The model under review builds one solid part; all positions refer to its coordinate system, in mm. A direction names the side the tool comes from. Coordinates: 2 decimals unless noted, no trailing zeros. Order: outer loops, then holes, each group sorted by start corner. A loop starts at its lowest first (then second) coordinate and runs counter-clockwise, first axis right, second up. Notation, with made-up numbers: (-18.5, 31.5) - (29.5, 31.5) arc R12 ccw to (29.5, 46.5) - close; hole circle Ø11 at (81, -3). An arc over 180 degrees is marked (long way). Answer in a Markdown table with one row per item.
```python
from build123d import *

# Parameters (mm, degrees)
F1_DEPTH  = 1
F4_W      = 25.4
F4_H      = 50.8
F5_DEPTH  = 34
F6_W      = 1.778
F6_H      = 3.81
F7_DEPTH  = 17.78
F8_W      = 20.32
F8_H      = 12.7
F9_DEPTH  = 7.62
F11_DEPTH = 25.4


with BuildPart() as f1:
    # F0 (on Top) → F1 (new body)
    with BuildSketch(Plane.XY):
        Polygon((12.7, 30), (0, 30), (0, 0), (20, 0), align=None)
    extrude(amount=F1_DEPTH)

    # F2: F1 across plane


with BuildPart() as f1_1:
    add(f1.part)
    add(f1.part.mirror(Plane.XZ))

    # F3: F1 across plane


with BuildPart() as f1_2:
    add(f1_1.part)
    add(f1_1.part.mirror(Plane.YZ))

    # F4 (on face) → F5 (join)
    with BuildSketch(Plane.XY.offset(1)):
        with Locations((-0.045811, 0)):
            Rectangle(F4_W, F4_H)
    extrude(amount=F5_DEPTH)

    # F6 (on face) → F7 (cut)
    with BuildSketch(Plane(origin=(0, 0, 0), x_dir=(1, 0, 0), z_dir=(0, 0, -1))):
        Polygon((-5.4, -22.54), (5, -22.54), (12.3, -15.24), (12.3, -2.54), (-12.7, -2.54), (-12.7, -15.24), align=None)
        with Locations((-5.969, -9.508814)):
            Rectangle(F6_W, F6_H, mode=Mode.SUBTRACT)
        with Locations((0.038805, -15.194196)):
            Rectangle(F6_W, F6_H, mode=Mode.SUBTRACT)
        with Locations((5.969, -9.508814)):
            Rectangle(F6_W, F6_H, mode=Mode.SUBTRACT)
    extrude(amount=-F7_DEPTH, mode=Mode.SUBTRACT)

    # F8 (on face) → F9 (join)
    with BuildSketch(Plane(origin=(0, 0, 0), x_dir=(1, 0, 0), z_dir=(0, 0, -1))):
        with Locations((0, 14.463713)):
            Rectangle(F8_W, F8_H)
    extrude(amount=F9_DEPTH)

    # F10 (on face) → F11 (cut)
    with BuildSketch(Plane(origin=(0, -8.113713, 0), x_dir=(-1, 0, 0), z_dir=(0, 1, 0))):
        Polygon((10.16, -7.62), (-10.16, -1.168574), (-10.16, -7.62), align=None)
        with BuildLine():
            ThreePointArc((10.16, -7.62), (0.686877, -2.230835), (-10.16, -1.168574))
            Line((-10.16, -1.168574), (10.16, -7.62))
        make_face()
    extrude(amount=-F11_DEPTH, mode=Mode.SUBTRACT)


solid = f1_2.part
```
Item 1: We need section D-D, the plane x = 8.5. Write out the cut boundary in (y, z), then the cut area to 3 significant figures.
Check values:
| item | result |
|---|---|
| outline | (-30, 0) - (-20.81, 0) - (-20.81, -1.03) - (-8.11, -1.03) - (-8.11, 0) - (2.54, 0) - (2.54, 17.78) - (19.04, 17.78) - (19.04, 0) - (30, 0) - (30, 1) - (25.4, 1) - (25.4, 35) - (-25.4, 35) - (-25.4, 1) - (-30, 1) - close |
| area | 1,510 mm^2 |
Item 2: We need section A-A, the plane z = 11. Write out the cut boundary in (x, y).
Check values:
| item | result |
|---|---|
| outline | (-12.75, -25.4) - (12.65, -25.4) - (12.65, 25.4) - (-12.75, 25.4) - close; (-6.86, 7.6) - (-5.08, 7.6) - (-5.08, 11.41) - (-6.86, 11.41) - close; (-0.85, 13.29) - (0.93, 13.29) - (0.93, 17.1) - (-0.85, 17.1) - close; (5.08, 7.6) - (6.86, 7.6) - (6.86, 11.41) - (5.08, 11.41) - close; hole (-12.7, 2.54) - (12.3, 2.54) - (12.3, 15.24) - (5, 22.54) - (-5.4, 22.54) - (-12.7, 15.24) - close |
Item 3: We need section B-B, the plane x = -12. Write out the cut boundary in (y, z).
Check values:
| item | result |
|---|---|
| outline | (-30, 0) - (2.54, 0) - (2.54, 17.78) - (15.94, 17.78) - (15.94, 0) - (30, 0) - (30, 1) - (25.4, 1) - (25.4, 35) - (-25.4, 35) - (-25.4, 1) - (-30, 1) - close |
Item 4: We need section C-C, the plane y = -12. Write out the cut boundary in (x, z).
Check values:
| item | result |
|---|---|
| outline | (-17.08, 0) - (-10.16, 0) - (-10.16, -7.62) arc R26.17 cw to (10.16, -1.17) - (10.16, 0) - (17.08, 0) - (17.08, 1) - (12.65, 1) - (12.65, 35) - (-12.75, 35) - (-12.75, 1) - (-17.08, 1) - close |
Item 5: Tool access review of faces 1 (the face through (0.928, 15, 9)), 2 (the face through (0, -25.4, 18)), 3 (the face through (-6, 9, 0)), 4 (the face through (0, 25.4, 18)): name each direction out of +Z, -Z, +X, -X, +Y, -Y from which nothing blocks a thin tool from reaching the whole face with its end or side.
Check values:
| item | result |
|---|---|
| face 1 | -Z |
| face 2 | +Z, +X, -X, -Y |
| face 3 | -Z, +X, -X, +Y |
| face 4 | +Z, +X, -X, +Y |
Item 6: Mouldability with a two-part tool opening along X and no side actions: class faces 5 (the face through (-5, -8.114, -2)), 6 (the face through (-10.16, -14, -4)), 7 (the face through (-9.1, 18.84, 8.77)) as +X half, -X half, draft (parallel to the pull), parting line (faces both ways), or undercut.
Check values:
| item | result |
|---|---|
| face 5 | draft |
| face 6 | -X half |
| face 7 | undercut |
Item 7: Clearance check with flat-ended pins moving along their axes: pin 1 Ø3 at (y, z) = (9, 11.5) entering from -X; pin 2 Ø20.5 at (x, z) = (-0.5, 23) entering from -Y; pin 3 Ø2 at (x, z) = (-0.5, 4.5) entering from +Y. State where each tip first meets the part, or that it passes through.
Check values:
| item | result |
|---|---|
| pin 1 | x = -12.75 |
| pin 2 | y = -25.4 |
| pin 3 | y = 25.4 |
Item 8: To check wall thickness, follow line 1 (Y direction, x = 6, z = 2); line 2 (X direction, y = -23.5, z = 24.5); line 3 (Y direction, x = 10, z = 24). State the ranges of each line that lie inside material, in increasing order. Write a range as from..to.
Check values:
| item | result |
|---|---|
| line 1 | -25.4..2.54, 7.6..11.41, 21.54..25.4 |
| line 2 | -12.75..12.65 |
| line 3 | -25.4..25.4 |
